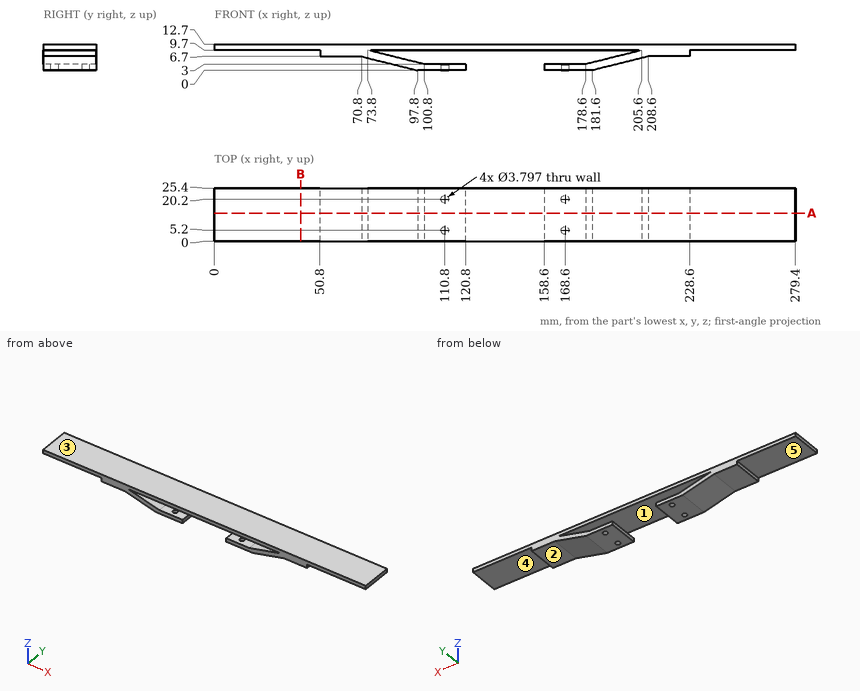
Study the drawing (mm; zero at the part's minimum x, y, z) and answer. A direction names the side the tool comes from. Coordinates: 2 decimals unless noted, no trailing zeros. Write each loop counter-clockwise with the first axis right and the second up, starting at its lowest first coordinate (ties: lowest second). Pieces come first, ordered by that corner, then holes. Notation, with made-up numbers: (-17.75, -9.5) - (32.25, -9.5) arc R24 ccw to (32.25, 6.5) - close; hole circle Ø10 at (56, -30). An arc over 180 degrees is marked (long way). Answer as a JSON object with one key per item and string values.
Q1. Which of the six approach directions +Z, -Z, +X, -X, +Y, -Y give full straight-line access (tool end or side, diameter ignored) to the marked faces 4 and 5?
Results list:
{"face 4": "-Z, +X, +Y, -Y", "face 5": "-Z, -X, +Y, -Y"}
Q2. For a pull along Z with two mould halves and no side action, classify the marked faces 1, 2 and 3 as pulls with the +Z half, pulls with the -Z half, needs draft (parallel to the pull), parting line crosses it, or undercut.
Results list:
{"face 1": "undercut", "face 2": "pulls with the -Z half", "face 3": "pulls with the +Z half"}
Q3. Given pin 1 Ø6 at (x, y) = (206.5, 20) entering from -Z; pin 2 Ø1.5 at (x, y) = (225.5, 16.5) entering from -Z; pin 3 Ø1.5 at (y, z) = (6.5, 8) entering from -X, each flat-ended and moving along its own axis, determine where each tip first touches the part or whether it passes through.
Results list:
{"pin 1": "stops at z = 5.43", "pin 2": "stops at z = 6.7", "pin 3": "stops at x = 50.8"}
Q4. Find section B-B (x = 41.5). Write down the section's boundary in (y, z), plus the area to 3 significant figures.
Results list:
{"outline": "(0, 9.7) - (25.4, 9.7) - (25.4, 12.7) - (0, 12.7) - close", "area": "76.2 mm^2"}
Q5. Consider L1, parallel to Y at x = 168.6, z = 1.45; L2, parallel to Z at x = 57, y = 23.5; L3, parallel to Z at x = 235, y = 16. Determine where each line is inside the solid, lowest interval first. Write a range as from..to.
Results list:
{"L1": "y = 0..3.3, 7.1..18.3, 22.1..25.4", "L2": "z = 6.7..12.7", "L3": "z = 9.7..12.7"}
Q6. Find section A-A (y = 13.5). Write down the section's boundary in (x, z).
Results list:
{"outline": "(0, 9.7) - (50.8, 9.7) - (50.8, 6.7) - (70.8, 6.7) - (97.8, 0) - (120.8, 0) - (120.8, 3) - (100.8, 3) - (73.8, 9.7) - (205.6, 9.7) - (178.6, 3) - (158.6, 3) - (158.6, 0) - (181.6, 0) - (208.6, 6.7) - (228.6, 6.7) - (228.6, 9.7) - (279.4, 9.7) - (279.4, 12.7) - (0, 12.7) - close"}
